Geometry check sheet. Reference: the model listing, model coordinates, mm. Coordinates: 2 decimals unless noted, no trailing zeros. Write each loop counter-clockwise with the first axis right and the second up, starting at its lowest first coordinate (ties: lowest second). Pieces come first, ordered by that corner, then holes.
from build123d import *

# Parameters (mm, degrees)
F0_R     = 38
F1_DEPTH = 4


with BuildPart() as f1:
    # F0 (on Right) → F1 (new body)
    with BuildSketch(Plane.YZ):
        Polygon((-180, 0), (0, 0), (504.79022, 971.705631), (-593.940286, 1024.538159), align=None)
        with Locations((-143, 50)):
            Circle(F0_R, mode=Mode.SUBTRACT)
        with Locations((-37, 50)):
            Circle(F0_R, mode=Mode.SUBTRACT)
    extrude(amount=F1_DEPTH)


solid = f1.part
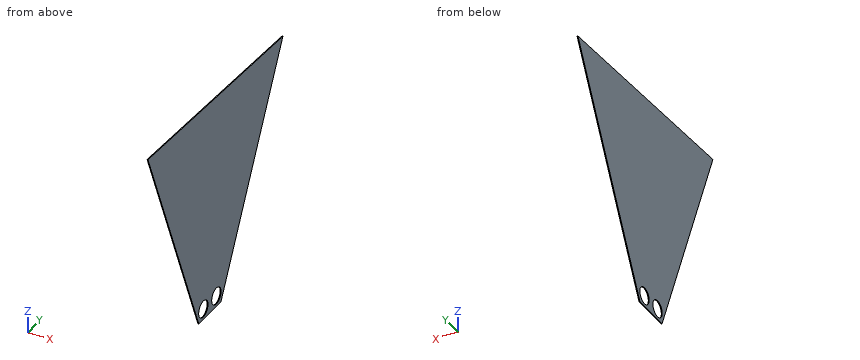
1. Sectioned sample at C-C, the plane z = 104.5. Record the boundary of the cut face in (x, y), and give its area (3 significant figures).
Computed values:
outline: (0, -222.22) - (4, -222.22) - (4, 54.29) - (0, 54.29) - close
area: 1,110 mm2
2. Gauge pin test, flat ends, axial feed: pin 1 Ø1 at (x, y) = (3, -257.5) entering from +Z; pin 2 Ø2 at (x, y) = (2.5, -230) entering from +Z; pin 3 Ø1.5 at (x, z) = (1, 604) entering from -Y. Record the tip position at first contact, or that the pin passes through.
Computed values:
pin 1: stops at z = 1008.38
pin 2: stops at z = 1007.09
pin 3: stops at y = -424.33
3. Sectioned sample at B-B, the plane x = 2.6. Record the boundary of the cut face in (y, z), and give its area (3 significant figures).
Computed values:
outline: (-593.94, 1024.54) - (-180, 0) - (0, 0) - (504.79, 971.71) - close; hole circle Ø76 at (-143, 50); hole circle Ø76 at (-37, 50)
area: 630,000 mm2
4. Sectioned sample at D-D, the plane y = -210. Record the boundary of the cut face in (x, z).
Computed values:
outline: (0, 74.25) - (4, 74.25) - (4, 1006.08) - (0, 1006.08) - close
5. Sectioned sample at A-A, the plane y = -33.5. Record the boundary of the cut face in (x, z).
Computed values:
outline: (0, 0) - (4, 0) - (4, 12.16) - (0, 12.16) - close; (0, 87.84) - (4, 87.84) - (4, 997.59) - (0, 997.59) - close
6. Thickness scan on line 1 along Z through (x, y) = (2.15, -143); line 2 along Z through (x, y) = (0.8, -37); line 3 along Z through (x, y) = (1.85, -517). Record the ranges inside material, lowest first.
Computed values:
line 1: z = 0 to 12, 88 to 1002.85
line 2: z = 0 to 12, 88 to 997.76
line 3: z = 834.1 to 1020.84
